For this review, take the finished solid that the model builds, in its own axes (mm). A direction names the side the tool comes from. Round coordinates to 2 decimals unless told otherwise and drop trailing zeros. Order: outer loops, then holes, each group sorted by start corner. A loop starts at its lowest first (then second) coordinate and runs counter-clockwise, first axis right, second up. Notation, with made-up numbers: M -29.75,83.5 L -4.75,83.5 A9 ccw -4.75,99.5 Z; hole C 8,61.5 d6. An arc over 180 degrees is marked long. Answer as a JSON object with one key per item and string values.
from build123d import *

# Parameters (mm, degrees)
ESQUISSE1_R                                    = 20
BOSS_EXTRU_1_DEPTH                             = 3
ESQUISSE2_R                                    = 11
BOSS_EXTRU_2_DEPTH                             = 3
CHANFREIN1_SIZE                                = 0.5
ESQUISSE3_R                                    = 7
ENL_V_MAT_EXTRU_1_DEPTH                        = 7
FRAISAGE_POUR_VIS_T_TE_FRAIS_E_M32_D           = 3.4
FRAISAGE_POUR_VIS_T_TE_FRAIS_E_M32_CSINK_D     = 6.3
FRAISAGE_POUR_VIS_T_TE_FRAIS_E_M32_CSINK_ANGLE = 90
R_P_TITION_CIRCULAIRE1_COUNT                   = 3


with BuildPart() as part:
    # Esquisse1 → Boss.-Extru.1 (new body)
    with BuildSketch(Plane.XY):
        Circle(ESQUISSE1_R)
    extrude(amount=BOSS_EXTRU_1_DEPTH)

    # Esquisse2 → Boss.-Extru.2 (add)
    with BuildSketch(Plane.XY.offset(3)):
        Circle(ESQUISSE2_R)
    extrude(amount=BOSS_EXTRU_2_DEPTH)

    # Chanfrein1
    chanfrein1_edges = [part.edges().sort_by_distance(p)[0] for p in [
        (-11, 0, 6),
    ]]
    chamfer(chanfrein1_edges, length=CHANFREIN1_SIZE)

    # Esquisse3 → Enlèv. mat.-Extru.1 (cut, through all)
    with BuildSketch(Plane(origin=(0, 0, 0), x_dir=(-1, 0, 0), z_dir=(0, 0, -1))):
        Circle(ESQUISSE3_R)
    extrude(amount=-ENL_V_MAT_EXTRU_1_DEPTH, mode=Mode.SUBTRACT)

    # Fraisage pour vis à tête fraisée M32 (through all)
    with Locations(Plane(origin=(0, 0, 0), x_dir=(-1, 0, 0), z_dir=(0, 0, -1))):
        with Locations((0, 15.5)):
            fraisage_pour_vis_t_te_frais_e_m32 = CounterSinkHole(FRAISAGE_POUR_VIS_T_TE_FRAIS_E_M32_D / 2, FRAISAGE_POUR_VIS_T_TE_FRAIS_E_M32_CSINK_D / 2, counter_sink_angle=FRAISAGE_POUR_VIS_T_TE_FRAIS_E_M32_CSINK_ANGLE)

    # Répétition circulaire1: Fraisage pour vis à tête fraisée M32 ×3 about axis
    r_p_tition_circulaire1_axis = Axis((0, 0, 0), (0, 0, 1))
    for i in range(1, R_P_TITION_CIRCULAIRE1_COUNT):
        add(fraisage_pour_vis_t_te_frais_e_m32.rotate(r_p_tition_circulaire1_axis, i * 360 / R_P_TITION_CIRCULAIRE1_COUNT), mode=Mode.SUBTRACT)


solid = part.part
1) Machinability: for faces 1 (the flat face through (9, -9, 3)), 2 (the cylindrical face through (14.208, -9.258, 2.236)), which of the approach directions +Z, -Z, +X, -X, +Y, -Y give a long, thin tool a straight path to every point of the face, cutting with its end or side? Answer none if there is none.
Geometry check:
{"face 1": "+Z", "face 2": "+Z, -Z"}
2) For L1, parallel to X at y = -7.75, z = 2.5; L2, parallel to Y at x = 0, z = 3.35; L3, parallel to Z at x = -18, y = -3.5, list the stretches that pass through material, from the lowest coordinate up.
Geometry check:
{"L1": "x = -18.44 to -15.12, -11.72 to 11.72, 15.12 to 18.44", "L2": "y = -11 to -7, 7 to 11", "L3": "z = 0 to 3"}
3) Add section D-D on y = -7.75. State how many separate pieces and enclosed holes the cut face has, and give its area (3 significant figures).
Geometry check:
{"separate pieces": "3", "enclosed holes": "0", "area": "132 mm²"}
4) Insertion check: P1, Ø4.5, axis at x = -13.42, y = -7.75, coming from the +Z side; P2, Ø1.5, axis at y = 3.5, z = 4, coming from the -X side; P3, Ø3, axis at x = 13.42, y = -7.75, coming from the +Z side. Each pin has a flat end and moves straight along its axis. Give the tip position at first contact, or say it passes through.
Geometry check:
{"P1": "stops at z = 3", "P2": "stops at x = -10.65", "P3": "passes through"}
5) Mouldability with a two-part tool opening along Y and no side actions: class faces 3 (the cylindrical face through (-0.37, 13.84, 2.24)), 4 (the cylindrical face through (-2.38, -10.74, 4.23)), 5 (the flat face through (2, -7, 6)) as +Y half, -Y half, draft (parallel to the pull), parting line (faces both ways), or undercut.
Geometry check:
{"face 3": "undercut", "face 4": "parting line", "face 5": "draft"}
6) Add section B-B on z = 0.5. State the section outline as (x, y) points, and give its area (3 significant figures).
Geometry check:
{"outline": "C 0,0 d40; hole C -13.42,-7.75 d5.3; hole C 0,0 d14; hole C 0,15.5 d5.3; hole C 13.42,-7.75 d5.3", "area": "1,040 mm²"}
7) Add section C-C on z = 4.4. State the section outline as (x, y) points, and give its area (3 significant figures).
Geometry check:
{"outline": "C 0,0 d22; hole C 0,0 d14", "area": "226 mm²"}
8) Add section A-A on y = 0. State the section outline as (x, z) points, and give its area (3 significant figures).
Geometry check:
{"outline": "M -20,0 L -7,0 L -7,6 L -10.5,6 L -11,5.5 L -11,3 L -20,3 Z; M 7,0 L 20,0 L 20,3 L 11,3 L 11,5.5 L 10.5,6 L 7,6 Z", "area": "102 mm²"}
